Autodesk Inventor part; units mm, degrees
ref_plane "YZ Plane" through (0, 0, 0) normal (1, 0, 0) x (0, 1, 0)
ref_plane "XZ Plane" through (0, 0, 0) normal (0, 1, 0) x (-1, 0, 0)
ref_plane "XY Plane" through (0, 0, 0) normal (0, 0, 1) x (1, 0, 0)
sketch "Sketch1" plane through (0, 0, 0) normal (0, 0, 1) x (1, 0, 0)
  line L0 (6.25, -22.5) -> (-8.25, -22.5)
  line L1 (-8.25, -22.5) -> (-8.25, 22.5)
  line L2 (-8.25, 22.5) -> (6.25, 22.5)
  line L3 (6.25, 22.5) -> (6.25, -22.5)
  line L4 (3.25, -12) -> (-3.25, -12)
  line L5 (-3.25, -12) -> (-3.25, 10)
  line L6 (-3.25, 10) -> (3.25, 10)
  line L7 (3.25, 10) -> (3.25, -12)
  line L8 (-11.15, 0) -> (9.15, 0)
  line L9 (0, -12) -> (0, 0) construction
  point P0 (6.25, 0)
  dimension "d0" = 6.5
  dimension "d3" = 45
  dimension "d10" = 3
  dimension "d11" = 5
  dimension "d25" = 10
  dimension "d26" = 12
extrude "Extrusion1" add sketch "Sketch1" along normal blind 1.5 contours L0 L1 L8 L5 L4 L7 L3 | L8 L7 L6 L5 L1 L2 L3
fillet "Fillet1" radius 2 4 edges at (6.25, 22.5, 0.75) (-8.25, 22.5, 0.75) (6.25, -22.5, 0.75) (-8.25, -22.5, 0.75)
chamfer "Chamfer1" distance 0.5 angle 45 4 edges at (3.25, -1, 0) (0, 10, 0) (-3.25, -1, 0) (0, -12, 0)
sketch "Sketch2" plane through (0, 0, 0) normal (0, 0, -1) x (-1, 0, 0)
  line L0 (4.65, -21.475) -> (-1.3, -21.475)
  line L1 (-3.3, -19.475) -> (-3.3, 19.475)
  line L2 (-1.3, 21.475) -> (4.65, 21.475)
  line L3 (6.65, 19.475) -> (6.65, -19.475)
  line L4 (3.25, 10) -> (3.25, -12)
  arc A0 (-3.3, -19.475) -> (-1.3, -21.475) centre (-1.3, -19.475) ccw
  arc A1 (4.65, -21.475) -> (6.65, -19.475) centre (4.65, -19.475) ccw
  arc A2 (6.65, 19.475) -> (4.65, 21.475) centre (4.65, 19.475) ccw
  arc A3 (-1.3, 21.475) -> (-3.3, 19.475) centre (-1.3, 19.475) ccw
  line L5 (-2.5, 19.475) -> (-2.5, -19.475)
  arc A4 (-2.5, -19.475) -> (-1.3, -20.675) centre (-1.3, -19.475) ccw
  line L6 (-1.3, -20.675) -> (4.65, -20.675)
  arc A5 (4.65, -20.675) -> (5.85, -19.475) centre (4.65, -19.475) ccw
  line L7 (5.85, -19.475) -> (5.85, 19.475)
  arc A6 (5.85, 19.475) -> (4.65, 20.675) centre (4.65, 19.475) ccw
  line L8 (4.65, 20.675) -> (-1.3, 20.675)
  arc A7 (-1.3, 20.675) -> (-2.5, 19.475) centre (-1.3, 19.475) ccw
  line L9 (-2.5, 12) -> (-3.3, 12)
  line L10 (-2.5, -14) -> (-3.3, -14)
  line L11 (3.25, -12) -> (-3.25, -12)
  line L12 (-3.25, 10) -> (3.25, 10)
  point P0 (0, 0)
  point P1 (-3.3, 21.475)
  point P2 (6.65, 21.475)
  dimension "d12" = 42.95
  dimension "d14" = 9.95
  dimension "d16" = 3.4
  dimension "d17" = 21.475
  dimension "d18" = 2
  dimension "d19" = 0.8
  dimension "d20" = 2
  dimension "d21" = 2
extrude "Extrusion2" add sketch "Sketch2" along normal blind 3 contours L0 A0 L1 L10 L5 A4 L6 A5 L7 A6 L8 A7 L9 A3 L2 A2 L3 A1
fillet "Fillet2" radius 0.4 4 edges at (3.3, -14, -1.5) (2.5, -14, -1.5) (3.3, 12, -1.5) (2.5, 12, -1.5)
equation "\"d21\" = d20"
properties part number "EndSwitchHousing_v02_TopPlate"
Geometry check sheet. Reference: the model listing, model coordinates, mm. A direction names the side the tool comes from. Give positions to 0.01 mm unless a question says otherwise; leave off trailing zeros. Order: outer loops, then holes, each group sorted by start corner. A loop starts at its lowest first (then second) coordinate and runs counter-clockwise, first axis right, second up.
1. Sectioned sample at C-C (y = -9.5). Record the boundary of the cut face in (x, z).
Completed:
outline: (-8.25, 0) - (-6.65, 0) - (-6.65, -3) - (-5.85, -3) - (-5.85, 0) - (-3.75, 0) - (-3.25, 0.5) - (-3.25, 1.5) - (-8.25, 1.5) - close; (3.25, 0.5) - (3.75, 0) - (6.25, 0) - (6.25, 1.5) - (3.25, 1.5) - close
2. Sectioned sample at B-B (z = 1.05). Record the boundary of the cut face in (x, y).
Completed:
outline: (-8.25, -20.5) arc R2 ccw to (-6.25, -22.5) - (4.25, -22.5) arc R2 ccw to (6.25, -20.5) - (6.25, 20.5) arc R2 ccw to (4.25, 22.5) - (-6.25, 22.5) arc R2 ccw to (-8.25, 20.5) - close; hole (-3.25, -12) - (3.25, -12) - (3.25, 10) - (-3.25, 10) - close
3. Depth check by flat-ended pin: pin 1 (0.9 mm diameter, centred on x = -2, z = -1, fed in from -Y) (3 decimals); pin 2 (1.5 mm diameter, centred on x = -2.5, z = -1.5, fed in from +Y) (3 decimals); pin 3 (1.5 mm diameter, centred on y = -17.5, z = -2, fed in from -X). Enter the tip coordinate at first touch or a pass-through.
Completed:
pin 1: stops at y = -21.475
pin 2: stops at y = 21.475
pin 3: stops at x = -6.65
4. Access from +Z, -Z, +X, -X, +Y, -Y to the whole of each face (thin tool, end or side, straight path). Record for faces 1 (the face through (0, 10, 1)), 2 (the face through (2.699, -20.905, -1.479)), 3 (the face through (3.3, -17, -1)), 4 (the face through (-2, 21.475, -1)).
Completed:
face 1: +Z, -Z
face 2: -Z, +X, -Y
face 3: -Z, +X, +Y, -Y
face 4: -Z, +X, -X, +Y
5. Draft check along X on faces 5 (the face through (-6, 5, -3)), 6 (the face through (5.65, -21.93, 0.76)), 7 (the face through (2.5, 16, -1)). Enter one of: pulls with the +X half, pulls with the -X half, needs draft (parallel to the pull), parting line crosses it, or undercut.
Completed:
face 5: needs draft
face 6: pulls with the +X half
face 7: undercut
6. Scan lines: line 1 (X direction, y = 5, z = 0.95); line 2 (X direction, y = -18, z = -0.15); line 3 (Y direction, x = -0.75, z = -0.6) (3 decimals). Record each from-to range of solid material in increasing order.
Completed:
line 1: x = -8.25 to -3.25, 3.25 to 6.25
line 2: x = -6.65 to -5.85, 2.5 to 3.3
line 3: y = -21.475 to -20.675, 20.675 to 21.475
7. Sectioned sample at A-A (x = -1.75). Record the boundary of the cut face in (y, z) (3 decimals), then the cut area to 4 significant figures.
Completed:
outline: (-22.5, 0) - (-21.475, 0) - (-21.475, -3) - (-20.675, -3) - (-20.675, 0) - (-12.5, 0) - (-12, 0.5) - (-12, 1.5) - (-22.5, 1.5) - close; (10, 0.5) - (10.5, 0) - (20.675, 0) - (20.675, -3) - (21.475, -3) - (21.475, 0) - (22.5, 0) - (22.5, 1.5) - (10, 1.5) - close
area: 39.05 mm2
8. Sectioned sample at D-D (y = -19). Record the boundary of the cut face in (x, z).
Completed:
outline: (-8.25, 0) - (-6.65, 0) - (-6.65, -3) - (-5.85, -3) - (-5.85, 0) - (2.5, 0) - (2.5, -3) - (3.3, -3) - (3.3, 0) - (6.25, 0) - (6.25, 1.5) - (-8.25, 1.5) - close
